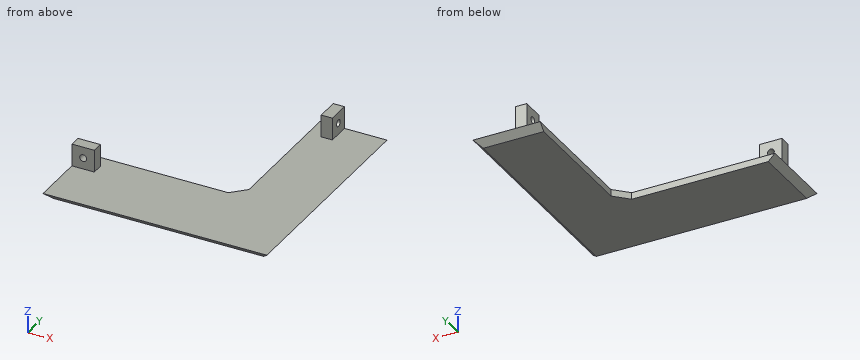
```python
from build123d import *

# Parameters (mm, degrees)
ESQUISSE1_W             = 100
ESQUISSE1_H             = 100
BOSS_EXTRU_1_DEPTH      = 3
CHANFREIN2_SIZE         = 3
ESQUISSE4_W             = 5
ESQUISSE4_H             = 10
ESQUISSE4_W_2           = 10
ESQUISSE4_H_2           = 5
BOSS_EXTRU_3_DEPTH      = 10
ESQUISSE5_R             = 1.525
ENL_V_MAT_EXTRU_2_DEPTH = 10
ESQUISSE6_R             = 1.525
ENL_V_MAT_EXTRU_3_DEPTH = 10
ESQUISSE7_W             = 70
ESQUISSE7_H             = 65
ENL_V_MAT_EXTRU_4_DEPTH = 10
CHANFREIN3_SIZE         = 6


with BuildPart() as part:
    # Esquisse1 → Boss.-Extru.1 (new body)
    with BuildSketch(Plane.XY):
        with Locations((50, 50)):
            Rectangle(ESQUISSE1_W, ESQUISSE1_H)
    extrude(amount=BOSS_EXTRU_1_DEPTH)

    # Chanfrein2
    chanfrein2_edges = [part.edges().sort_by_distance(p)[0] for p in [
        (50, 0, 0),
        (100, 50, 0),
        (50, 100, 0),
        (0, 50, 0),
    ]]
    chamfer(chanfrein2_edges, length=CHANFREIN2_SIZE - 0.0001)  # a hair under: the kernel refuses the full size

    # Esquisse4 → Boss.-Extru.3 (add)
    with BuildSketch(Plane.XY.offset(3)):
        with Locations((78.5, 94.95)):
            Rectangle(ESQUISSE4_W, ESQUISSE4_H)
        with Locations((5.05, 26.5)):
            Rectangle(ESQUISSE4_W_2, ESQUISSE4_H_2)
    extrude(amount=BOSS_EXTRU_3_DEPTH)

    # Esquisse5 → Enlèv. mat.-Extru.2 (cut)
    with BuildSketch(Plane(origin=(81, 0, 0), x_dir=(0, 0, -1), z_dir=(1, 0, 0))):
        with Locations((-8.05, 94.95)):
            Circle(ESQUISSE5_R)
    extrude(amount=-ENL_V_MAT_EXTRU_2_DEPTH, mode=Mode.SUBTRACT)

    # Esquisse6 → Enlèv. mat.-Extru.3 (cut)
    with BuildSketch(Plane(origin=(0, 29, 0), x_dir=(1, 0, 0), z_dir=(0, 1, 0))):
        with Locations(Location((5.05, -8, 0), (0, 0, 270))):
            Circle(ESQUISSE6_R)
    extrude(amount=-ENL_V_MAT_EXTRU_3_DEPTH, mode=Mode.SUBTRACT)

    # Esquisse7 → Enlèv. mat.-Extru.4 (cut)
    with BuildSketch(Plane.XY.offset(3)):
        with Locations((35, 67.5)):
            Rectangle(ESQUISSE7_W, ESQUISSE7_H)
    extrude(amount=-ENL_V_MAT_EXTRU_4_DEPTH, mode=Mode.SUBTRACT)

    # Chanfrein3
    chanfrein3_edges = [part.edges().sort_by_distance(p)[0] for p in [
        (70, 35, 1.5),
    ]]
    chamfer(chanfrein3_edges, length=CHANFREIN3_SIZE)


solid = part.part
```
For this review, take the finished solid that the model builds, in its own axes (mm). Give positions to 0.01 mm unless a question says otherwise; leave off trailing zeros. Order: outer loops, then holes, each group sorted by start corner. A loop starts at its lowest first (then second) coordinate and runs counter-clockwise, first axis right, second up.
1) Take a section at C-C (z = 8.05). Give the boundary of the cut face in (x, y) (3 decimals), then the cut area to 3 significant figures.
2) Insertion check: pin 1 (2.5 mm diameter, centred on y = 26.5, z = 6, fed in from +X); pin 2 (1.5 mm diameter, centred on x = 79, z = 6, fed in from +Y); pin 3 (3.5 mm diameter, centred on x = 5.05, z = 8, fed in from -Y). Each pin has a flat end and moves straight along its axis. Give the tip position at first contact, or say it passes through.
3) Wall thickness on line 1 (Z direction, x = 77.85, y = 94.95) (3 decimals); line 2 (Y direction, x = 79.25, z = 8.05) (3 decimals); line 3 (X direction, y = 27.9, z = 8) (3 decimals): over which ranges is each line inside the solid? List them lowest first.
Derived:
1. outline: (0.05, 24) - (3.526, 24) - (3.526, 29) - (0.05, 29) - close; (6.574, 24) - (10.05, 24) - (10.05, 29) - (6.574, 29) - close; (76, 89.95) - (81, 89.95) - (81, 93.425) - (76, 93.425) - close; (76, 96.475) - (81, 96.475) - (81, 99.95) - (76, 99.95) - close
1. area: 69.5 mm2
2. pin 1: stops at x = 10.05
2. pin 2: stops at y = 99.95
2. pin 3: stops at y = 24
3. line 1: z = 0 to 6.525, 9.575 to 13
3. line 2: y = 89.95 to 93.425, 96.475 to 99.95
3. line 3: x = 0.05 to 3.525, 6.575 to 10.05
